Verification items for the finished model (mm, model axes). A direction names the side the tool comes from. Round coordinates to 2 decimals unless told otherwise and drop trailing zeros. Loops run counter-clockwise (first coordinate to the right, second up) from the corner with the lowest first, then second, coordinate; pieces in that order, holes last. Notation, with made-up numbers: (81, 64.5) -> (137, 64.5) arc R23 cw to (137, 78.5) -> close; hole circle Ø10 at (48, -19). An arc over 180 degrees is marked (long way). Write item = value, one per line. Start each with the question number.
```python
from build123d import *

# Parameters (mm, degrees)
SKETCH_1_R      = 1
EXTRUDE_1_DEPTH = 1


with BuildPart() as part:
    # 草图1 → 凸台-拉伸1 (new body)
    with BuildSketch(Plane(origin=(0, 0, 0), x_dir=(1, 0, 0), z_dir=(0, 1, 0))):
        with BuildLine():
            Line((-2, 16.38774479), (-2, 15.88774479))
            ThreePointArc((-2, 15.88774479), (-1.646446609, 15.034191399), (-2.5, 15.38774479))
            Line((-2.5, 15.38774479), (-3, 15.38774479))
            Line((-3, 15.38774479), (-3, 14.38774479))
            Line((-3, 14.38774479), (-3, 3.38774479))
            Line((-3, 3.38774479), (-3, 2.087766192))
            Line((-3, 2.087766192), (-3, 0.887766192))
            Line((-3, 0.887766192), (-2.5, 0.887766192))
            ThreePointArc((-2.5, 0.887766192), (-1.646446609, 1.241319582), (-2, 0.387766192))
            Line((-2, 0.387766192), (-2, -0.312233808))
            Line((-2, -0.312233808), (2, -0.312233808))
            Line((2, -0.312233808), (2, 0.387766192))
            ThreePointArc((2, 0.387766192), (1.646446609, 1.241319582), (2.5, 0.887766192))
            Line((2.5, 0.887766192), (3, 0.887766192))
            Line((3, 0.887766192), (3, 2.087766192))
            Line((3, 2.087766192), (3, 3.38774479))
            Line((3, 3.38774479), (3, 14.38774479))
            Line((3, 14.38774479), (3, 15.38774479))
            Line((3, 15.38774479), (2.5, 15.38774479))
            ThreePointArc((2.5, 15.38774479), (1.646446609, 15.034191399), (2, 15.88774479))
            Line((2, 15.88774479), (2, 16.58774479))
            Line((2, 16.58774479), (-2, 16.58774479))
            Line((-2, 16.58774479), (-2, 16.38774479))
        make_face()
        with BuildLine():
            ThreePointArc((1.238170819, 2.380547047), (-0.011829181, 1.130547047), (-1.261829181, 2.380547047))
            Line((-1.261829181, 2.380547047), (-1.261829181, 7.380547047))
            ThreePointArc((-1.261829181, 7.380547047), (-0.011829181, 8.630547047), (1.238170819, 7.380547047))
            Line((1.238170819, 7.380547047), (1.238170819, 2.380547047))
        make_face(mode=Mode.SUBTRACT)
        with Locations(Location((-0.011829181, 10.562782389, 0), (0, 0, 270))):
            Circle(SKETCH_1_R, mode=Mode.SUBTRACT)
        with BuildLine():
            ThreePointArc((0.988170819, 13.456705927), (-0.011829181, 12.456705927), (-1.011829181, 13.456705927))
            Line((-1.011829181, 13.456705927), (-1.011829181, 14.456705927))
            ThreePointArc((-1.011829181, 14.456705927), (-0.011829181, 15.456705927), (0.988170819, 14.456705927))
            Line((0.988170819, 14.456705927), (0.988170819, 13.456705927))
        make_face(mode=Mode.SUBTRACT)
    extrude(amount=EXTRUDE_1_DEPTH)


solid = part.part
```
(1) Draft check along X on faces 1 (the cylindrical face through (-0.04, 0.49, -8.63)), 2 (the flat face through (0, 0.5, -16.588)), 3 (the flat face through (-3, 0.5, -8.2)). Enter one of: +X half, -X half, draft (parallel to the pull), parting line (faces both ways), or undercut.
(2) Section check A-A on x = 1.75. Enter the section's corners in (y, z).
(3) Section check D-D on y = 0.5. Enter the section's corners in (x, z).
(4) Access from +Z, -Z, +X, -X, +Y, -Y to the whole of each face (thin tool, end or side, straight path). Record for faces 4 (the flat face through (-1.262, 0.5, -4.8)), 5 (the flat face through (3, 0.5, -8)).
(5) Scan lines: line 1 (Z direction, x = 0.05, y = 0.6); line 2 (X direction, y = 0.2, z = -5); line 3 (Z direction, x = -0.9, y = 0.6). Record each from-to range of solid material in increasing order. Write a range as [from, to].
(6) Section check C-C on x = 0.75. Enter the section's corners in (y, z) (3 decimals).
(7) Section check B-B on z = -11. Enter the section's corners in (x, y).
Computed values:
q1.face_1 = undercut
q1.face_2 = draft
q1.face_3 = -X half
q2.outline = (0, -16.59) -> (1, -16.59) -> (1, -15.82) -> (0, -15.82) -> close; (0, -14.95) -> (1, -14.95) -> (1, -1.32) -> (0, -1.32) -> close; (0, -0.45) -> (1, -0.45) -> (1, 0.31) -> (0, 0.31) -> close
q3.outline = (-3, -15.39) -> (-2.5, -15.39) arc R0.5 cw (long way) to (-2, -15.89) -> (-2, -16.59) -> (2, -16.59) -> (2, -15.89) arc R0.5 cw (long way) to (2.5, -15.39) -> (3, -15.39) -> (3, -0.89) -> (2.5, -0.89) arc R0.5 cw (long way) to (2, -0.39) -> (2, 0.31) -> (-2, 0.31) -> (-2, -0.39) arc R0.5 cw (long way) to (-2.5, -0.89) -> (-3, -0.89) -> close; hole (-1.26, -7.38) arc R1.25 ccw to (1.24, -7.38) -> (1.24, -2.38) arc R1.25 ccw to (-1.26, -2.38) -> close; hole (-1.01, -14.46) arc R1 ccw to (0.99, -14.46) -> (0.99, -13.46) arc R1 ccw to (-1.01, -13.46) -> close; hole circle Ø2 at (-0.01, -10.56)
q4.face_4 = +Y, -Y
q4.face_5 = +Z, -Z, +X, +Y, -Y
q5.line_1 = [-16.59, -15.45], [-12.46, -11.56], [-9.56, -8.63], [-1.13, 0.31]
q5.line_2 = [-3, -1.26], [1.24, 3]
q5.line_3 = [-16.59, -14.92], [-13, -11.02], [-10.1, -8.26], [-1.5, 0.31]
q6.outline = (0, -16.588) -> (1, -16.588) -> (1, -15.104) -> (0, -15.104) -> close; (0, -12.809) -> (1, -12.809) -> (1, -11.211) -> (0, -11.211) -> close; (0, -9.915) -> (1, -9.915) -> (1, -8.372) -> (0, -8.372) -> close; (0, -1.39) -> (1, -1.39) -> (1, 0.312) -> (0, 0.312) -> close
q7.outline = (-3, 0) -> (-0.91, 0) -> (-0.91, 1) -> (-3, 1) -> close; (0.89, 0) -> (3, 0) -> (3, 1) -> (0.89, 1) -> close
